from build123d import *

# Parameters (mm, degrees)
AUFSATZ_LINEAR_AUSTRAGEN1_DEPTH = 3


with BuildPart() as part:
    # Skizze1 → Aufsatz-Linear austragen1 (new body)
    with BuildSketch(Plane(origin=(0, 0, 0), x_dir=(1, 0, 0), z_dir=(0, 1, 0))):
        Polygon((4.885929648, 7.801507538), (4.885929648, 0.301507538), (7.985929648, 0.301507538), (7.985929648, 7.801507538), (21.385929648, 7.801507538), (21.385929648, 0.301507538), (24.485929648, 0.301507538), (24.485929648, 7.801507538), (37.885929648, 7.801507538), (37.885929648, 0.301507538), (40.985929648, 0.301507538), (40.985929648, 7.801507538), (54.385929648, 7.801507538), (54.385929648, 0.301507538), (57.485929648, 0.301507538), (57.485929648, 7.801507538), (70.885929648, 7.801507538), (70.885929648, 0.301507538), (73.985929648, 0.301507538), (73.985929648, 7.801507538), (87.385929648, 7.801507538), (87.385929648, 0.301507538), (90.485929648, 0.301507538), (90.485929648, 7.801507538), (103.885929648, 7.801507538), (103.885929648, 0.301507538), (106.985929648, 0.301507538), (106.985929648, 7.801507538), (120.385929648, 7.801507538), (120.385929648, 0.301507538), (123.485929648, 0.301507538), (123.485929648, 7.801507538), (136.885929648, 7.801507538), (136.885929648, 0.301507538), (139.985929648, 0.301507538), (139.985929648, 7.801507538), (153.385929648, 7.801507538), (153.385929648, 0.301507538), (156.485929648, 0.301507538), (156.485929648, 7.801507538), (169.885929648, 7.801507538), (169.885929648, 0.301507538), (172.985929648, 0.301507538), (172.985929648, 7.801507538), (186.385929648, 7.801507538), (186.385929648, 0.301507538), (189.485929648, 0.301507538), (189.485929648, 7.801507538), (202.885929648, 7.801507538), (202.885929648, 0.301507538), (205.985929648, 0.301507538), (205.985929648, 7.801507538), (222.185929648, 7.801507538), (222.185929648, -7.198492462), (-27.814070352, -7.198492462), (-27.814070352, 7.801507538), (-11.614070352, 7.801507538), (-11.614070352, 0.301507538), (-8.514070352, 0.301507538), (-8.514070352, 7.801507538), align=None)
    extrude(amount=AUFSATZ_LINEAR_AUSTRAGEN1_DEPTH)


solid = part.part
The listing builds one solid part. Answer for the finished solid, in the listing's coordinates (mm). Give positions to 0.01 mm unless a question says otherwise; leave off trailing zeros. One line per item, written item: value. Start each with the question number.
1) Find the intervals of material crossed by L1, parallel to Z at x = 188.5, y = 1.1, in increasing order.
2) Given pin 1 Ø2 at (x, z) = (164, 4) entering from -Y, flat-ended and moving along its own axis, determine where the tip first touches the part or whether it passes through.
3) A cutting plane is placed at A-A on z = -5.75. State how many separate pieces and enclosed holes the cut face has, then the cut area to 3 significant figures.
Answer sheet:
1. L1: z = -0.3 to 7.2
2. pin 1: stops at y = 0
3. separate pieces: 15
3. enclosed holes: 0
3. area: 620 mm2
